Part model, mm, in its own coordinate system. A direction names the side the tool comes from. Round coordinates to 2 decimals unless told otherwise and drop trailing zeros. Order: outer loops, then holes, each group sorted by start corner. A loop starts at its lowest first (then second) coordinate and runs counter-clockwise, first axis right, second up. Notation, with made-up numbers: (-4.75, 7.5) -> (3.25, 7.5) arc R26 ccw to (3.25, 21.5) -> close; hole circle Ø7 at (61.5, 21.5). An arc over 180 degrees is marked (long way). Return JSON: item names as keys, results as strings. Group by question number.
from build123d import *

# Parameters (mm, degrees)
SKETCH1_W                 = 90
SKETCH1_H                 = 35
SKETCH1_R                 = 14.2875
SKETCH1_R_2               = 4.5
BOSS_EXTRUDE1_DEPTH       = 6.5278
SKETCH2_W                 = 20
SKETCH2_H                 = 35
SKETCH2_R                 = 4.5
BOSS_EXTRUDE2_DEPTH       = 44.45
BOSS_EXTRUDE3_OUTLINE_W   = 90
BOSS_EXTRUDE3_OUTLINE_H   = 35
BOSS_EXTRUDE3_OUTLINE_R   = 1.984375
BOSS_EXTRUDE3_OUTLINE_R_2 = 6.35
BOSS_EXTRUDE3_OUTLINE_R_3 = 4.5
BOSS_EXTRUDE3_DEPTH       = 6.5278


# Read off the part's stored shape, not the designer's step: Boss-Extrude3
with BuildPart() as part:
    # Sketch1 → Boss-Extrude1 (new body)
    with BuildSketch(Plane(origin=(0, 0, 0), x_dir=(0, 0, -1), z_dir=(1, 0, 0))):
        with Locations((10, 0)):
            Rectangle(SKETCH1_W, SKETCH1_H)
        with Locations(Location((0, 0, 0), (0, 0, 180))):
            Circle(SKETCH1_R, mode=Mode.SUBTRACT)
        with Locations(Location((45, 4, 0), (0, 0, 180))):
            Circle(SKETCH1_R_2, mode=Mode.SUBTRACT)
    extrude(amount=BOSS_EXTRUDE1_DEPTH)

    # Sketch2 → Boss-Extrude2 (add)
    with BuildSketch(Plane(origin=(6.5278, 0, 0), x_dir=(0, 0, -1), z_dir=(1, 0, 0))):
        with Locations((45, 0)):
            Rectangle(SKETCH2_W, SKETCH2_H)
        with Locations(Location((45, 4, 0), (0, 0, 180))):
            Circle(SKETCH2_R, mode=Mode.SUBTRACT)
    extrude(amount=BOSS_EXTRUDE2_DEPTH)

    # Boss-Extrude3 outline → Boss-Extrude3 (add)
    with BuildSketch(Plane(origin=(50.9778, 0, 0), x_dir=(0, 0, -1), z_dir=(1, 0, 0))):
        with Locations((10, 0)):
            Rectangle(BOSS_EXTRUDE3_OUTLINE_W, BOSS_EXTRUDE3_OUTLINE_H)
        with Locations((-25.4, 0)):
            Circle(BOSS_EXTRUDE3_OUTLINE_R, mode=Mode.SUBTRACT)
        Circle(BOSS_EXTRUDE3_OUTLINE_R_2, mode=Mode.SUBTRACT)
        with Locations((25.4, 0)):
            Circle(BOSS_EXTRUDE3_OUTLINE_R, mode=Mode.SUBTRACT)
        with Locations((45, 4)):
            Circle(BOSS_EXTRUDE3_OUTLINE_R_3, mode=Mode.SUBTRACT)
    extrude(amount=BOSS_EXTRUDE3_DEPTH)


solid = part.part
(1) Probe L1, parallel to X at y = 8, z = 22; L2, parallel to Y at x = 3, z = 0; L3, parallel to X at y = -7.5, z = -3. List the from-to ranges inside material, lowest first. Write a range as [from, to].
(2) Saw through at C-C, the plane z = 25.4. List the corners of the cut face in (x, y), and give its area (3 significant figures).
(3) Saw through at B-B, the plane x = 38. List the corners of the cut face in (y, z), and give its area (3 significant figures).
(4) Saw through at A-A, the plane z = -45. List the corners of the cut face in (x, y).
(5) Saw through at D-D, the plane y = -11.5. List the corners of the cut face in (x, z).
(6) Tool access for faces 1 (the flat face through (28, 0, -35)), 2 (the cylindrical face through (54.196, -1.207, 26.975)), 3 (the cylindrical face through (3.218, -0.628, -14.274)), 4 (the flat face through (0, 0, -19)), 5 (the flat face through (54, 0, 35)): list every direction of +Z, -Z, +X, -X, +Y, -Y with a clear straight run to the whole face (end or side of a thin tool).
(7) Pin check, flat tips, straight feed: P1, Ø17, axis at y = 0, z = 0, coming from the -X side; P2, Ø3.5, axis at y = 0, z = -25.4, coming from the +X side; P3, Ø17.5, axis at x = 23, y = 2, coming from the +Z side. Stop position of each tip, or through.
(8) Mould opens along Y. For faces 6 (the cylindrical face through (54.196, -1.207, -23.825)), 7 (the flat face through (28, -17.5, -39)), 8 (the flat face through (28, 17.5, -39)), 9 (the flat face through (6.528, 11.9, 8.3)) say: pulls with the +Y half, pulls with the -Y half, needs draft (parallel to the pull), parting line crosses it, or undercut.
Results are:
{
 "1": {"L1": "x = [0, 6.53], [50.98, 57.51]", "L2": "y = [-17.5, -14.29], [14.29, 17.5]", "L3": "x = [50.98, 57.51]"},
 "2": {"outline": "(0, -17.5) -> (6.53, -17.5) -> (6.53, 17.5) -> (0, 17.5) -> close; (50.98, -17.5) -> (57.51, -17.5) -> (57.51, -1.98) -> (50.98, -1.98) -> close; (50.98, 1.98) -> (57.51, 1.98) -> (57.51, 17.5) -> (50.98, 17.5) -> close", "area": "431 mm^2"},
 "3": {"outline": "(-17.5, -55) -> (17.5, -55) -> (17.5, -35) -> (-17.5, -35) -> close; hole circle Ø9 at (4, -45)", "area": "636 mm^2"},
 "4": {"outline": "(0, -17.5) -> (57.51, -17.5) -> (57.51, -0.5) -> (0, -0.5) -> close; (0, 8.5) -> (57.51, 8.5) -> (57.51, 17.5) -> (0, 17.5) -> close"},
 "5": {"outline": "(0, -55) -> (57.51, -55) -> (57.51, 35) -> (50.98, 35) -> (50.98, -35) -> (6.53, -35) -> (6.53, -8.48) -> (0, -8.48) -> close; (0, 8.48) -> (6.53, 8.48) -> (6.53, 35) -> (0, 35) -> close"},
 "6": {"face 1": "+Z, +Y, -Y", "face 2": "+X", "face 3": "-X", "face 4": "+Z, -Z, -X, +Y, -Y", "face 5": "+Z, +X, -X, +Y, -Y"},
 "7": {"P1": "stops at x = 50.98", "P2": "stops at x = 6.53", "P3": "stops at z = -35"},
 "8": {"face 6": "undercut", "face 7": "pulls with the -Y half", "face 8": "pulls with the +Y half", "face 9": "needs draft"}
}
